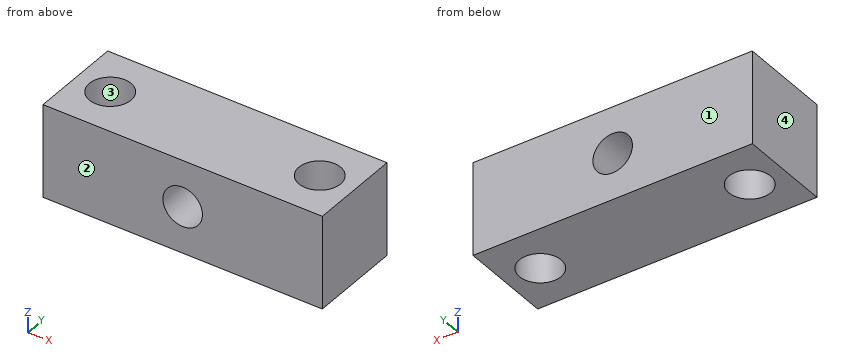
from build123d import *

# Parameters (mm, degrees)
SKETCH_1_W              = 60
SKETCH_1_H              = 20
SKETCH_1_R              = 4.5
EXTRUDE_1_DEPTH         = 20
HOLE_WIZARD_M10_1_D     = 8.5
HOLE_WIZARD_M10_1_DEPTH = 24.5
HOLE_WIZARD_M10_1_TIP   = 2.553657631


with BuildPart() as part:
    # 草图1 → 凸台-拉伸1 (new body)
    with BuildSketch(Plane.XY):
        Rectangle(SKETCH_1_W, SKETCH_1_H)
        with Locations((-22.5, 0)):
            Circle(SKETCH_1_R, mode=Mode.SUBTRACT)
        with Locations((22.5, 0)):
            Circle(SKETCH_1_R, mode=Mode.SUBTRACT)
    extrude(amount=EXTRUDE_1_DEPTH)

    # M10 螺纹孔1
    with Locations(Plane(origin=(0, 10, 10), x_dir=(0, 0, 1), z_dir=(0, 1, 0))):
        with Locations((0, 0)):
            Hole(HOLE_WIZARD_M10_1_D / 2, depth=HOLE_WIZARD_M10_1_DEPTH)
            with Locations((0, 0, -(HOLE_WIZARD_M10_1_DEPTH + HOLE_WIZARD_M10_1_TIP / 2))):  # 118° drill point
                Cone(0, HOLE_WIZARD_M10_1_D / 2, HOLE_WIZARD_M10_1_TIP, mode=Mode.SUBTRACT)


solid = part.part
Can you work these out from the model? Positions are in its coordinate system, mm. Face numbers are marked on the shaded views. Give positions to 0.01 mm unless a question says otherwise; leave off trailing zeros. Order: outer loops, then holes, each group sorted by start corner. A loop starts at its lowest first (then second) coordinate and runs counter-clockwise, first axis right, second up. Notation, with made-up numbers: M 13.5,-12 L 53.5,-12 A6 ccw 53.5,-3 Z; hole C 8,-1 d11. An arc over 180 degrees is marked long. Use a Markdown table: item, result. Add a question column.
Item 1: Suppose I cut it at B-B (y = 0). List the corners of the cut face in (x, z) for me, then the cut area to 3 significant figures.
Item 2: Will these pins go through, and if not, where does the flat tip stop? pin 1 (5 mm diameter, centred on x = 3, z = 10, fed in from +Y); pin 2 (5.5 mm diameter, centred on x = -22.5, y = 0, fed in from -Z).
Item 3: Suppose I cut it at A-A (x = -22.5). List the corners of the cut face in (y, z) for me.
Item 4: Suppose I cut it at C-C (z = 10). List the corners of the cut face in (x, y) for me, then the cut area to 3 significant figures.
Item 5: If I drill on L1, parallel to Y at x = 22.5, z = 11.25; L2, parallel to X at y = 3.75, z = 15.75; L3, parallel to X at y = -8, z = 10, over which ranges is the centre line in solid material (lowest first)? Write a range as [from, to].
Item 6: Suppose I cut it at D-D (y = 8.5). List the corners of the cut face in (x, z) for me.
Item 7: We'd pull the mould along Y, two halves only. Please class the marked faces 1, 2, 3 and 4: +Y half, -Y half, draft (parallel to the pull), parting line (faces both ways), or undercut.
Answer sheet:
| question | item | result |
|---|---|---|
| 1 | outline | M -30,0 L -27,0 L -27,20 L -30,20 Z; M -18,0 L 18,0 L 18,20 L -18,20 Z; M 27,0 L 30,0 L 30,20 L 27,20 Z; hole C 0,10 d8.5 |
| 1 | area | 783 mm² |
| 2 | pin 1 | stops at y = 10 |
| 2 | pin 2 | passes through |
| 3 | outline | M -10,0 L -4.5,0 L -4.5,20 L -10,20 Z; M 4.5,0 L 10,0 L 10,20 L 4.5,20 Z |
| 4 | outline | M -30,-10 L -4.25,-10 L -4.25,10 L -30,10 Z; M 4.25,-10 L 30,-10 L 30,10 L 4.25,10 Z; hole C -22.5,0 d9; hole C 22.5,0 d9 |
| 4 | area | 903 mm² |
| 5 | L1 | y = [-10, -4.5], [4.5, 10] |
| 5 | L2 | x = [-30, -24.99], [-20.01, 20.01], [24.99, 30] |
| 5 | L3 | x = [-30, -4.25], [4.25, 30] |
| 6 | outline | M -30,0 L 30,0 L 30,20 L -30,20 Z; hole C 0,10 d8.5 |
| 7 | face 1 | +Y half |
| 7 | face 2 | -Y half |
| 7 | face 3 | undercut |
| 7 | face 4 | draft |
